Design review of the part built by this model. Coordinates are the model's own, in mm. A direction names the side the tool comes from. Give positions to 0.01 mm unless a question says otherwise; leave off trailing zeros. Loops run counter-clockwise (first coordinate to the right, second up) from the corner with the lowest first, then second, coordinate; pieces in that order, holes last. Notation, with made-up numbers: M 63,34.5 L 117,34.5 A21 ccw 117,62.5 Z; hole C 33,77.5 d3. An arc over 180 degrees is marked long. Use CSV: the item, a comma, the result in double quotes.
from build123d import *

# Parameters (mm, degrees)
SKETCH1_R           = 2.19
SKETCH1_R_2         = 2.5
SKETCH1_R_3         = 1.5
BOSS_EXTRUDE1_DEPTH = 6.35


with BuildPart() as part:
    # Sketch1 → Boss-Extrude1 (new body)
    with BuildSketch(Plane(origin=(0, 0, 0), x_dir=(1, 0, 0), z_dir=(0, 1, 0))):
        with BuildLine():
            Line((-9.153018436, -1.431925443), (-66.073018436, -1.431925443))
            Line((-66.073018436, -1.431925443), (-75.073018436, -1.431925443))
            Line((-75.073018436, -1.431925443), (-75.073018436, -6.511925443))
            Line((-75.073018436, -6.511925443), (-75.073018436, -29.251925443))
            Line((-75.073018436, -29.251925443), (-75.073018436, -34.331925443))
            Line((-75.073018436, -34.331925443), (-66.073018436, -34.331925443))
            Line((-66.073018436, -34.331925443), (-9.153018436, -34.331925443))
            ThreePointArc((-9.153018436, -34.331925443), (-5.560915987, -32.844027891), (-4.073018436, -29.251925443))
            Line((-4.073018436, -29.251925443), (-4.073018436, -6.511925443))
            ThreePointArc((-4.073018436, -6.511925443), (-5.560915987, -2.919822995), (-9.153018436, -1.431925443))
        make_face()
        with Locations(Location((-57.593170924, -22.966925443, 0), (0, 0, 270))):
            Circle(SKETCH1_R, mode=Mode.SUBTRACT)
        with Locations(Location((-57.593170924, -12.796925443, 0), (0, 0, 90))):
            Circle(SKETCH1_R, mode=Mode.SUBTRACT)
        with Locations(Location((-10.093170924, -12.796925443, 0), (0, 0, 270))):
            Circle(SKETCH1_R, mode=Mode.SUBTRACT)
        with Locations(Location((-69.991443077, -17.881925443, 0), (0, 0, 270))):
            Circle(SKETCH1_R_2, mode=Mode.SUBTRACT)
        with Locations(Location((-10.093170924, -22.966925443, 0), (0, 0, 90))):
            Circle(SKETCH1_R_3, mode=Mode.SUBTRACT)
        Polygon((-13.903170924, -18.881925443), (-13.903170924, -27.791925443), (-54.003170924, -27.791925443), (-54.003170924, -18.881925443), (-62.003170924, -18.881925443), (-62.003170924, -16.881925443), (-54.003170924, -16.881925443), (-54.003170924, -7.971925443), (-13.903170924, -7.971925443), (-13.903170924, -16.881925443), (-6.073018436, -16.881925443), (-6.073018436, -18.881925443), align=None, mode=Mode.SUBTRACT)
    extrude(amount=BOSS_EXTRUDE1_DEPTH)


solid = part.part
(1) We need section A-A on z = 26. State the section outline as (x, y) points, then the cut area to 3 significant figures.
A:
outline,"M -75.07,0 L -54,0 L -54,6.35 L -75.07,6.35 Z; M -13.9,0 L -4.07,0 L -4.07,6.35 L -13.9,6.35 Z"
area,"196 mm²"
(2) We need section B-B on x = -19. State the section outline as (y, z) points, then the cut area to 3 significant figures.
A:
outline,"M 0,1.43 L 6.35,1.43 L 6.35,7.97 L 0,7.97 Z; M 0,27.79 L 6.35,27.79 L 6.35,34.33 L 0,34.33 Z"
area,"83.1 mm²"
(3) We need section C-C on y = 3. State the section outline as (x, z) points.
A:
outline,"M -75.07,1.43 L -9.15,1.43 A5.08 ccw -4.07,6.51 L -4.07,29.25 A5.08 ccw -9.15,34.33 L -75.07,34.33 Z; hole C -69.99,17.88 d5; hole M -62,16.88 L -54,16.88 L -54,7.97 L -13.9,7.97 L -13.9,16.88 L -6.07,16.88 L -6.07,18.88 L -13.9,18.88 L -13.9,27.79 L -54,27.79 L -54,18.88 L -62,18.88 Z; hole C -57.59,12.8 d4.38; hole C -57.59,22.97 d4.38; hole C -10.09,12.8 d4.38; hole C -10.09,22.97 d3"
(4) Wall thickness on line 1 along Z through (x, y) = (-47, 5.75); line 2 along Z through (x, y) = (-11, 4); line 3 along X through (y, z) = (6.25, 21): over which ranges is each line inside the solid? List them lowest first. Write a range as [from, to].
A:
line 1,"[1.43, 7.97], [27.79, 34.33]"
line 2,"[1.43, 10.8], [14.79, 16.88], [18.88, 21.77], [24.16, 34.33]"
line 3,"[-75.07, -58.56], [-56.63, -54], [-13.9, -4.07]"
(5) Machinability: for faces 1 (the flat face through (-4.073, 3, 18)), 2 (the flat face through (-13.903, 3, 12)), which of the approach directions +Z, -Z, +X, -X, +Y, -Y give a long, thin tool a straight path to every point of the face, cutting with its end or side? Answer none if there is none.
A:
face 1,"+Z, -Z, +X, +Y, -Y"
face 2,"+Y, -Y"
(6) The part is to be moulded in two halves that separate along Z. For faces 3 (the flat face through (-6.073, 3, 18)), 4 (the flat face through (-13.903, 3, 23)), 5 (the cylindrical face through (-5.52, 3.13, 2.96)), 6 (the flat face through (-43, 3, 34.332)), say which applies: released by +Z, released by -Z, zero draft, split by the parting line, or undercut.
A:
face 3,"undercut"
face 4,"undercut"
face 5,"released by -Z"
face 6,"released by +Z"
